Check sheet for the modelled part. Datum: model origin and axes. Units: mm. Face numbers are marked on the shaded views. Round coordinates to 2 decimals unless told otherwise and drop trailing zeros. Loops run counter-clockwise (first coordinate to the right, second up) from the corner with the lowest first, then second, coordinate; pieces in that order, holes last. Notation, with made-up numbers: (31, -30) - (39, -30) arc R25 cw to (39, 0) - close; hole circle Ø8 at (17, -16). An arc over 180 degrees is marked (long way). Put each result on its own line as item: value.
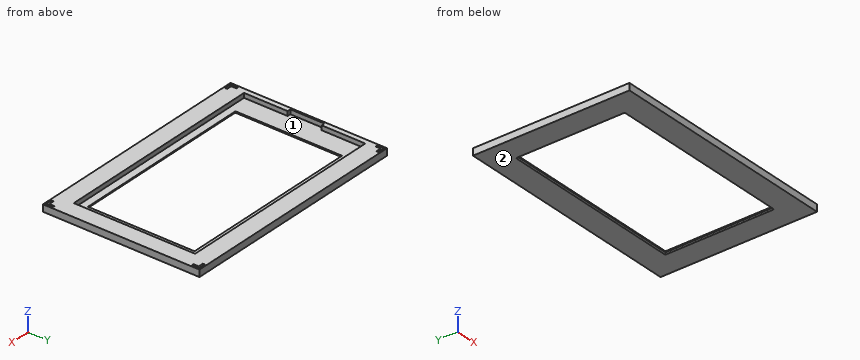
```python
from build123d import *

# Parameters (mm, degrees)
SKETCH1_W           = 103
SKETCH1_H           = 69
BOSS_EXTRUDE1_DEPTH = 3
SKETCH2_W           = 81
SKETCH2_H           = 47
CUT_EXTRUDE1_DEPTH  = 3
CUT_EXTRUDE2_DEPTH  = 2
CHAMFER1_SIZE       = 0.5
FILLET1_R           = 0.5
CUT_EXTRUDE3_DEPTH  = 1.1


with BuildPart() as part:
    # Sketch1 → Boss-Extrude1 (new body)
    with BuildSketch(Plane.XY):
        with Locations((62.328366078, 28.443882797)):
            Rectangle(SKETCH1_W, SKETCH1_H)
    extrude(amount=BOSS_EXTRUDE1_DEPTH)

    # Sketch2 → Cut-Extrude1 (cut)
    with BuildSketch(Plane.XY.offset(3)):
        with Locations((62.328366078, 28.443882797)):
            Rectangle(SKETCH2_W, SKETCH2_H)
    extrude(amount=-CUT_EXTRUDE1_DEPTH, mode=Mode.SUBTRACT)

    # Sketch3 → Cut-Extrude2 (cut)
    with BuildSketch(Plane.XY.offset(3)):
        Polygon((13.078366078, 55.193882797), (106.578366078, 55.193882797), (106.578366078, 1.693882797), (13.078366078, 1.693882797), (13.078366078, 20.943882797), (11.578366078, 20.943882797), (11.578366078, 35.943882797), (13.078366078, 35.943882797), align=None)
    extrude(amount=-CUT_EXTRUDE2_DEPTH, mode=Mode.SUBTRACT)

    # Chamfer1
    chamfer1_edges = [part.edges().sort_by_distance(p)[0] for p in [
        (21.828366078, 28.443882797, 0),
        (62.328366078, 51.943882797, 0),
        (102.828366078, 28.443882797, 0),
        (62.328366078, 4.943882797, 0),
    ]]
    chamfer(chamfer1_edges, length=CHAMFER1_SIZE)

    # Fillet1
    fillet1_edges = [part.edges().sort_by_distance(p)[0] for p in [
        (21.578366078, 52.193882797, 0.25),
        (103.078366078, 52.193882797, 0.25),
        (21.578366078, 4.693882797, 0.25),
        (103.078366078, 4.693882797, 0.25),
    ]]
    fillet(fillet1_edges, radius=FILLET1_R)

    # Sketch4 → Cut-Extrude3 (cut)
    with BuildSketch(Plane.XY.offset(3)):
        Polygon((11.503366078, 62.268882797), (14.653366078, 62.268882797), (14.653366078, 61.368882797), (12.403366078, 61.368882797), (12.403366078, 59.118882797), (11.503366078, 59.118882797), align=None)
        Polygon((113.153366078, 59.118882797), (113.153366078, 62.268882797), (110.003366078, 62.268882797), (110.003366078, 61.368882797), (112.253366078, 61.368882797), (112.253366078, 59.118882797), align=None)
        Polygon((113.153366078, -5.381117203), (110.003366078, -5.381117203), (110.003366078, -4.481117203), (112.253366078, -4.481117203), (112.253366078, -2.231117203), (113.153366078, -2.231117203), align=None)
        Polygon((11.503366078, -2.231117203), (11.503366078, -5.381117203), (14.653366078, -5.381117203), (14.653366078, -4.481117203), (12.403366078, -4.481117203), (12.403366078, -2.231117203), align=None)
    extrude(amount=-CUT_EXTRUDE3_DEPTH, mode=Mode.SUBTRACT)


solid = part.part
```
Item 1: Section check A-A on y = 24. Enter the section's corners in (x, z), then the cut area to 4 significant figures.
Filled sheet:
outline: (10.83, 0) - (21.33, 0) - (21.83, 0.5) - (21.83, 1) - (11.58, 1) - (11.58, 3) - (10.83, 3) - close; (102.83, 0.5) - (103.33, 0) - (113.83, 0) - (113.83, 3) - (106.58, 3) - (106.58, 1) - (102.83, 1) - close
area: 37.75 mm²
Item 2: Go/stop test with a flat-tipped pin: pin 1 (8 mm diameter, centred on x = 45.5, y = 48, fed in from -Z). Record where the tip stops, or that it passes through.
Filled sheet:
pin 1: z = 0.44
Item 3: Section check B-B on x = 43. Enter the section's corners in (y, z).
Filled sheet:
outline: (-6.06, 0) - (4.44, 0) - (4.94, 0.5) - (4.94, 1) - (1.69, 1) - (1.69, 3) - (-6.06, 3) - close; (51.94, 0.5) - (52.44, 0) - (62.94, 0) - (62.94, 3) - (55.19, 3) - (55.19, 1) - (51.94, 1) - close
Item 4: Release check for a two-part mould opening along X. For the marked faces 1 and 2 record: +X half, -X half, draft (parallel to the pull), parting line (faces both ways), or undercut.
Filled sheet:
face 1: undercut
face 2: draft
Item 5: Thickness scan on line 1 (Y direction, x = 35, z = 1.4); line 2 (X direction, y = 12, z = 2.7); line 3 (X direction, y = 33, z = 0.8). Record the ranges inside material, lowest first. Write a range as from..to.
Filled sheet:
line 1: -6.06..1.69, 55.19..62.94
line 2: 10.83..13.08, 106.58..113.83
line 3: 10.83..21.83, 102.83..113.83
